Here's how the part is built. I have some questions about the finished solid (model axes, mm). Face numbers are marked on the shaded views. A direction names the side the tool comes from. Round coordinates to 2 decimals unless told otherwise and drop trailing zeros. Order: outer loops, then holes, each group sorted by start corner. A loop starts at its lowest first (then second) coordinate and runs counter-clockwise, first axis right, second up.
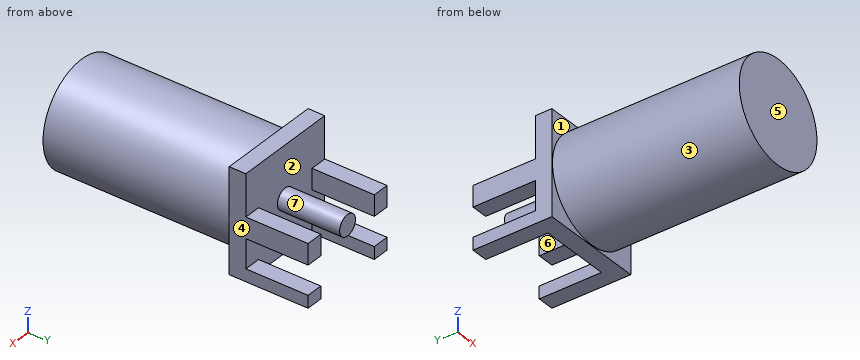
```python
from build123d import *

# Parameters (mm, degrees)
SKETCH1_W           = 6.35
SKETCH1_H           = 6.35
BOSS_EXTRUDE1_DEPTH = 1.02
SKETCH2_W           = 1.02
SKETCH2_H           = 0.76
SKETCH2_H_2         = 1.27
BOSS_EXTRUDE2_DEPTH = 3.81
SKETCH3_R           = 0.635
BOSS_EXTRUDE3_DEPTH = 3.81
SKETCH4_R           = 3.13
BOSS_EXTRUDE4_DEPTH = 11.43


with BuildPart() as part:
    # Sketch1 → Boss-Extrude1 (new body)
    with BuildSketch(Plane(origin=(0, 0, 0), x_dir=(1, 0, 0), z_dir=(0, 1, 0))):
        Rectangle(SKETCH1_W, SKETCH1_H)
    extrude(amount=BOSS_EXTRUDE1_DEPTH)

    # Sketch2 → Boss-Extrude2 (add)
    with BuildSketch(Plane(origin=(0, 1.02, 0), x_dir=(1, 0, 0), z_dir=(0, 1, 0))):
        with Locations((-2.665, 2.795)):
            Rectangle(SKETCH2_W, SKETCH2_H)
        with Locations((-2.665, 0.005)):
            Rectangle(SKETCH2_W, SKETCH2_H_2)
        with Locations((2.665, 0.005)):
            Rectangle(SKETCH2_W, SKETCH2_H_2)
        with Locations((2.665, 2.795)):
            Rectangle(SKETCH2_W, SKETCH2_H)
    extrude(amount=BOSS_EXTRUDE2_DEPTH)

    # Sketch3 → Boss-Extrude3 (add)
    with BuildSketch(Plane(origin=(0, 1.02, 0), x_dir=(1, 0, 0), z_dir=(0, 1, 0))):
        Circle(SKETCH3_R)
    extrude(amount=BOSS_EXTRUDE3_DEPTH)

    # Sketch4 → Boss-Extrude4 (add)
    with BuildSketch(Plane.XZ):
        Circle(SKETCH4_R)
    extrude(amount=BOSS_EXTRUDE4_DEPTH)


solid = part.part
```
1. I need wall thicknesses on probe 1 along X at (y, z) = (2.5, 0.25) (3 decimals); probe 2 along Y at (x, z) = (2.25, -1.25); probe 3 along Z at (x, y) = (-2, -2.75). Which ranges of each line are inside material? Lowest first, please.
Evaluation:
probe 1: x = -3.175 to -2.155, -0.584 to 0.584, 2.155 to 3.175
probe 2: y = -11.43 to 1.02
probe 3: z = -2.41 to 2.41
2. If we section it at D-D, the plane y = -3.25: Write out the boundary of the cut face in (x, z).
Evaluation:
outline: circle Ø6.26 at (0, 0)
3. I'm going to push flat-ended pins straight in: P1, Ø0.8, axis at x = 3, y = 3.5, coming from the +Z side; P2, Ø3, axis at y = -4.5, z = -1.5, coming from the +X side; P3, Ø1, axis at x = 1, y = -5, coming from the -Z side. Where does each tip first touch, or does it pass through?
Evaluation:
P1: stops at z = 0.63
P2: stops at x = 3.13
P3: stops at z = -3.09
4. If we section it at A-A, the plane y = 2: Write out the boundary of the cut face in (x, z) (3 decimals).
Evaluation:
outline: (-3.175, -3.175) - (-2.155, -3.175) - (-2.155, -2.415) - (-3.175, -2.415) - close; (-3.175, -0.64) - (-2.155, -0.64) - (-2.155, 0.63) - (-3.175, 0.63) - close; circle Ø1.27 at (0, 0); (2.155, -3.175) - (3.175, -3.175) - (3.175, -2.415) - (2.155, -2.415) - close; (2.155, -0.64) - (3.175, -0.64) - (3.175, 0.63) - (2.155, 0.63) - close
5. If we section it at C-C, the plane z = -1.25: Write out the boundary of the cut face in (x, y) (3 decimals).
Evaluation:
outline: (-3.175, 0) - (-2.87, 0) - (-2.87, -11.43) - (2.87, -11.43) - (2.87, 0) - (3.175, 0) - (3.175, 1.02) - (-3.175, 1.02) - close
6. On a 3-axis mill with a long thin cutter (end or side, diameter ignored), from which of +Z, -Z, +X, -X, +Y, -Y can I reach the whole of each face in a straight line? I mean the marked faces 5, 6 and 7. Say none if no direction works.
Evaluation:
face 5: +Z, -Z, +X, -X, -Y
face 6: +Z, -Z, +Y
face 7: +Y
7. If we mould it in two halves opening along X, with no side actions, what happens to the marked faces 1, 2, 3 and 4? For each: released by +X, released by -X, zero draft, split by the parting line, or undercut.
Evaluation:
face 1: zero draft
face 2: undercut
face 3: split by the parting line
face 4: released by +X
8. If we section it at B-B, the plane x = 0: Write out the boundary of the cut face in (y, z) (3 decimals), and give its area (3 significant figures).
Evaluation:
outline: (-11.43, -3.13) - (0, -3.13) - (0, -3.175) - (1.02, -3.175) - (1.02, -0.635) - (4.83, -0.635) - (4.83, 0.635) - (1.02, 0.635) - (1.02, 3.175) - (0, 3.175) - (0, 3.13) - (-11.43, 3.13) - close
area: 82.9 mm2
